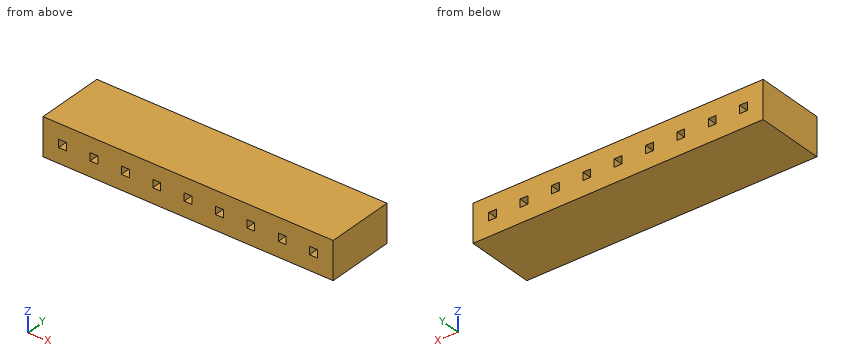
```python
from build123d import *

# Parameters (mm, degrees)
SKETCH1_W           = 18.5
SKETCH1_H           = 2.4
BOSS_EXTRUDE1_DEPTH = 4.37
SKETCH2_W           = 0.5
SKETCH2_H           = 0.5
CUT_EXTRUDE1_DEPTH  = 4.37


with BuildPart() as part:
    # Sketch1 → Boss-Extrude1 (new body)
    with BuildSketch(Plane(origin=(0, 0, 0), x_dir=(1, 0, 0), z_dir=(0, 1, 0))):
        with Locations((9, 1)):
            Rectangle(SKETCH1_W, SKETCH1_H)
    extrude(amount=BOSS_EXTRUDE1_DEPTH)

    # Sketch2 → Cut-Extrude1 (cut)
    with BuildSketch(Plane(origin=(0, 4.37, 0), x_dir=(1, 0, 0), z_dir=(0, 1, 0))):
        with Locations((3, 1)):
            Rectangle(SKETCH2_W, SKETCH2_H)
        with Locations((1, 1)):
            Rectangle(SKETCH2_W, SKETCH2_H)
        with Locations((5, 1)):
            Rectangle(SKETCH2_W, SKETCH2_H)
        with Locations((7, 1)):
            Rectangle(SKETCH2_W, SKETCH2_H)
        with Locations((9, 1)):
            Rectangle(SKETCH2_W, SKETCH2_H)
        with Locations((11, 1)):
            Rectangle(SKETCH2_W, SKETCH2_H)
        with Locations((13, 1)):
            Rectangle(SKETCH2_W, SKETCH2_H)
        with Locations((15, 1)):
            Rectangle(SKETCH2_W, SKETCH2_H)
        with Locations((17, 1)):
            Rectangle(SKETCH2_W, SKETCH2_H)
    extrude(amount=-CUT_EXTRUDE1_DEPTH, mode=Mode.SUBTRACT)


solid = part.part
```
Could you check a few things on this model? Use its own coordinates, in mm. Round coordinates to 2 decimals unless told otherwise and drop trailing zeros. Loops run counter-clockwise (first coordinate to the right, second up) from the corner with the lowest first, then second, coordinate; pieces in that order, holes last. Notation, with made-up numbers: (83.5, 47.25) - (117.5, 47.25) arc R6 cw to (117.5, 53.25) - close; hole circle Ø5 at (83, 48). An arc over 180 degrees is marked (long way). Answer in a Markdown table with one row per item. Add a question column.
(1) If we section it at A-A (x = 13): Please give me the cut outline in (y, z).
(2) I need wall thicknesses on line 1 along Z through (x, y) = (7, 2.6). Which ranges of the line are inside material? Lowest first, please.
(3) If we section it at B-B (y = 3.1): State how many separate pieces and enclosed holes the cut face has, plus the area to 4 significant figures.
Model answer:
| question | item | result |
|---|---|---|
| 1 | outline | (0, -2.2) - (4.37, -2.2) - (4.37, -1.25) - (0, -1.25) - close; (0, -0.75) - (4.37, -0.75) - (4.37, 0.2) - (0, 0.2) - close |
| 2 | line 1 | z = -2.2 to -1.25, -0.75 to 0.2 |
| 3 | separate pieces | 1 |
| 3 | enclosed holes | 9 |
| 3 | area | 42.15 mm² |
